Build history of the part. All positions in model axes, mm. A direction names the side the tool comes from. Round coordinates to 2 decimals unless told otherwise and drop trailing zeros. Write each loop counter-clockwise with the first axis right and the second up, starting at its lowest first coordinate (ties: lowest second). Pieces come first, ordered by that corner, then holes. Notation, with made-up numbers: (53, 24.25) -> (102, 24.25) arc R22 ccw to (102, 41.25) -> close; hole circle Ø9 at (9, 41.25). An arc over 180 degrees is marked (long way). Answer as CSV lines item,"result".
Solid Edge part; units mm, degrees
sketch "Sketch1" plane through (0, 0, 0) normal (0, 0, 1) x (1, 0, 0)
  circle A0 centre (0, 0) radius 3.175
extrude "Protrusion1" add sketch "Sketch1" along normal blind 6.35
chamfer "Chamfer1" distance 0.4762 angle 45 2 edges at (-3.175, 0, 0) (-3.175, 0, 6.35)
sketch "Sketch2" plane through (0, 0, 6.35) normal (0, 0, 1) x (1, 0, 0)
  line L0 (-0.9165, 1.5875) -> (0.9165, 1.5875)
  line L1 (1.8331, 0) -> (0.9165, 1.5875)
  line L2 (0.9165, -1.5875) -> (1.8331, 0)
  line L3 (-0.9165, -1.5875) -> (0.9165, -1.5875)
  line L4 (-1.8331, 0) -> (-0.9165, -1.5875)
  line L5 (-0.9165, 1.5875) -> (-1.8331, 0)
extrude "Cutout1" cut sketch "Sketch2" against normal blind 3.175
properties part number "24100599"
1. Cut at D-D, the plane z = 2.75. Write the cut outline in (x, y) (3 decimals), then the cut area to 3 significant figures.
Results found:
outline,"circle Ø6.35 at (0, 0)"
area,"31.7 mm2"
2. Probe line 1 along X through (y, z) = (-2.75, 5.75); line 2 along Z through (x, y) = (-1.25, 0) (3 decimals); line 3 along Y through (x, z) = (-1, 4.5). List the from-to ranges inside material, lowest first.
Results found:
line 1,"x = -1.59 to 1.59"
line 2,"z = 0 to 3.175"
line 3,"y = -3.01 to -1.44, 1.44 to 3.01"
3. Mould opens along X. For faces 1 (the flat face through (0, 1.588, 5)), 2 (the flat face through (0, 0, 0)), 3 (the cylindrical face through (-0.69, 3.1, 3.14)) say: +X half, -X half, draft (parallel to the pull), parting line (faces both ways), or undercut.
Results found:
face 1,"undercut"
face 2,"draft"
face 3,"parting line"
4. Drop a flat-ended pin along its axis: pin 1 Ø1 at (x, y) = (0.5, 0.5) entering from +Z (3 decimals). Give the stop position or say it passes through.
Results found:
pin 1,"stops at z = 3.175"
5. Cut at C-C, the plane z = 6.25. Write the cut outline in (x, y), then the cut area to 3 significant figures.
Results found:
outline,"circle Ø5.6 at (0, 0); hole (-1.83, 0) -> (-0.92, -1.59) -> (0.92, -1.59) -> (1.83, 0) -> (0.92, 1.59) -> (-0.92, 1.59) -> close"
area,"15.9 mm2"
6. Which spindle directions (+Z, -Z, +X, -X, +Y, -Y) get a long thin tool onto all of the face, cutting with end or side? Do faces 4 (the flat face through (0, -2, 6.35)), 5 (the flat face through (0, 0, 3.175)). Say none if no direction does.
Results found:
face 4,"+Z, +X, -X, +Y, -Y"
face 5,"+Z"
